```python
from build123d import *

# Parameters (mm, degrees)
CYLINDER1845_R     = 17
CYLINDER1845_DEPTH = 160
CYLINDER1789_R     = 4
CYLINDER1789_DEPTH = 100
CYLINDER1790_R     = 4
CYLINDER1790_DEPTH = 100
CYLINDER1809_R     = 1.5
CYLINDER1809_DEPTH = 100
CYLINDER1825_R     = 1.5
CYLINDER1825_DEPTH = 100
CYLINDER1824_R     = 1.5
CYLINDER1824_DEPTH = 100
CYLINDER1806_R     = 1.5
CYLINDER1806_DEPTH = 100
CYLINDER1805_R     = 1.5
CYLINDER1805_DEPTH = 100
CYLINDER1804_R     = 1.5
CYLINDER1804_DEPTH = 100
CYLINDER1803_R     = 1.5
CYLINDER1803_DEPTH = 100
CYLINDER1828_R     = 1.5
CYLINDER1828_DEPTH = 100
CYLINDER1826_R     = 4
CYLINDER1826_DEPTH = 100
CYLINDER1788_R     = 4
CYLINDER1788_DEPTH = 100
CYLINDER1787_R     = 4
CYLINDER1787_DEPTH = 100
CYLINDER1783_R     = 4
CYLINDER1783_DEPTH = 100
CYLINDER1785_R     = 4
CYLINDER1785_DEPTH = 100
CYLINDER1784_R     = 4
CYLINDER1784_DEPTH = 100
CYLINDER1786_R     = 4
CYLINDER1786_DEPTH = 100
CYLINDER1827_R     = 4
CYLINDER1827_DEPTH = 100
CYLINDER1797_R     = 4
CYLINDER1797_DEPTH = 20
CYLINDER1796_R     = 4
CYLINDER1796_DEPTH = 20
CYLINDER1795_R     = 4
CYLINDER1795_DEPTH = 20
CYLINDER1794_R     = 4
CYLINDER1794_DEPTH = 40
CYLINDER1793_R     = 4
CYLINDER1793_DEPTH = 40
CYLINDER1792_R     = 4
CYLINDER1792_DEPTH = 40
CYLINDER1791_R     = 4
CYLINDER1791_DEPTH = 40
CYLINDER1817_R     = 4
CYLINDER1817_DEPTH = 20
CYLINDER1798_R     = 59
CYLINDER1798_DEPTH = 16
CHAMFER061_SIZE    = 4
FILLET025_R        = 4


with BuildPart() as obj1:
    # Cylinder1845 → Cylinder1845 (new body)
    with BuildSketch(Plane(origin=(-18, 0, -60), x_dir=(1, 0, 0), z_dir=(0, 0, 1))):
        Circle(CYLINDER1845_R)
    extrude(amount=CYLINDER1845_DEPTH)


with BuildPart() as obj2:
    # Cylinder1789 → Cylinder1789 (new body)
    with BuildSketch(Plane(origin=(14, 0, -18), x_dir=(1, 0, 0), z_dir=(0, 0, 1))):
        Circle(CYLINDER1789_R)
    extrude(amount=CYLINDER1789_DEPTH)


with BuildPart() as obj3:
    # Cylinder1790 → Cylinder1790 (new body)
    with BuildSketch(Plane(origin=(90, 0, -18), x_dir=(1, 0, 0), z_dir=(0, 0, 1))):
        Circle(CYLINDER1790_R)
    extrude(amount=CYLINDER1790_DEPTH)

    # Compound957: union obj2
    add(obj2.part)


with BuildPart() as obj4:
    # Cylinder1809 → Cylinder1809 (new body)
    with BuildSketch(Plane(origin=(-34, -16, -60), x_dir=(1, 0, 0), z_dir=(0, 0, 1))):
        Circle(CYLINDER1809_R)
    extrude(amount=CYLINDER1809_DEPTH)


with BuildPart() as obj5:
    # Cylinder1825 → Cylinder1825 (new body)
    with BuildSketch(Plane(origin=(34, -16, -60), x_dir=(1, 0, 0), z_dir=(0, 0, 1))):
        Circle(CYLINDER1825_R)
    extrude(amount=CYLINDER1825_DEPTH)


with BuildPart() as obj6:
    # Cylinder1824 → Cylinder1824 (new body)
    with BuildSketch(Plane(origin=(34, 16, -60), x_dir=(1, 0, 0), z_dir=(0, 0, 1))):
        Circle(CYLINDER1824_R)
    extrude(amount=CYLINDER1824_DEPTH)


with BuildPart() as obj7:
    # Cylinder1806 → Cylinder1806 (new body)
    with BuildSketch(Plane(origin=(16, 34, -60), x_dir=(1, 0, 0), z_dir=(0, 0, 1))):
        Circle(CYLINDER1806_R)
    extrude(amount=CYLINDER1806_DEPTH)


with BuildPart() as obj8:
    # Cylinder1805 → Cylinder1805 (new body)
    with BuildSketch(Plane(origin=(10, -36, -60), x_dir=(1, 0, 0), z_dir=(0, 0, 1))):
        Circle(CYLINDER1805_R)
    extrude(amount=CYLINDER1805_DEPTH)


with BuildPart() as obj9:
    # Cylinder1804 → Cylinder1804 (new body)
    with BuildSketch(Plane(origin=(-16, -34, -60), x_dir=(1, 0, 0), z_dir=(0, 0, 1))):
        Circle(CYLINDER1804_R)
    extrude(amount=CYLINDER1804_DEPTH)


with BuildPart() as obj10:
    # Cylinder1803 → Cylinder1803 (new body)
    with BuildSketch(Plane(origin=(-16, 34, -60), x_dir=(1, 0, 0), z_dir=(0, 0, 1))):
        Circle(CYLINDER1803_R)
    extrude(amount=CYLINDER1803_DEPTH)


with BuildPart() as obj11:
    # Cylinder1828 → Cylinder1828 (new body)
    with BuildSketch(Plane(origin=(-34, 16, -60), x_dir=(1, 0, 0), z_dir=(0, 0, 1))):
        Circle(CYLINDER1828_R)
    extrude(amount=CYLINDER1828_DEPTH)

    # Compound954: union obj4, obj5, obj6, obj7, obj8, obj9, obj10
    add(obj4.part)
    add(obj5.part)
    add(obj6.part)
    add(obj7.part)
    add(obj8.part)
    add(obj9.part)
    add(obj10.part)


with BuildPart() as obj12:
    # Cylinder1826 → Cylinder1826 (new body)
    with BuildSketch(Plane(origin=(-16, 34, -90), x_dir=(1, 0, 0), z_dir=(0, 0, 1))):
        Circle(CYLINDER1826_R)
    extrude(amount=CYLINDER1826_DEPTH)


with BuildPart() as obj13:
    # Cylinder1788 → Cylinder1788 (new body)
    with BuildSketch(Plane(origin=(-16, -34, -90), x_dir=(1, 0, 0), z_dir=(0, 0, 1))):
        Circle(CYLINDER1788_R)
    extrude(amount=CYLINDER1788_DEPTH)


with BuildPart() as obj14:
    # Cylinder1787 → Cylinder1787 (new body)
    with BuildSketch(Plane(origin=(34, -16, -90), x_dir=(1, 0, 0), z_dir=(0, 0, 1))):
        Circle(CYLINDER1787_R)
    extrude(amount=CYLINDER1787_DEPTH)


with BuildPart() as obj15:
    # Cylinder1783 → Cylinder1783 (new body)
    with BuildSketch(Plane(origin=(16, 34, -90), x_dir=(1, 0, 0), z_dir=(0, 0, 1))):
        Circle(CYLINDER1783_R)
    extrude(amount=CYLINDER1783_DEPTH)


with BuildPart() as obj16:
    # Cylinder1785 → Cylinder1785 (new body)
    with BuildSketch(Plane(origin=(10, -36, -90), x_dir=(1, 0, 0), z_dir=(0, 0, 1))):
        Circle(CYLINDER1785_R)
    extrude(amount=CYLINDER1785_DEPTH)


with BuildPart() as obj17:
    # Cylinder1784 → Cylinder1784 (new body)
    with BuildSketch(Plane(origin=(-34, 16, -90), x_dir=(1, 0, 0), z_dir=(0, 0, 1))):
        Circle(CYLINDER1784_R)
    extrude(amount=CYLINDER1784_DEPTH)


with BuildPart() as obj18:
    # Cylinder1786 → Cylinder1786 (new body)
    with BuildSketch(Plane(origin=(34, 16, -90), x_dir=(1, 0, 0), z_dir=(0, 0, 1))):
        Circle(CYLINDER1786_R)
    extrude(amount=CYLINDER1786_DEPTH)


with BuildPart() as obj19:
    # Cylinder1827 → Cylinder1827 (new body)
    with BuildSketch(Plane(origin=(-34, -16, -90), x_dir=(1, 0, 0), z_dir=(0, 0, 1))):
        Circle(CYLINDER1827_R)
    extrude(amount=CYLINDER1827_DEPTH)

    # Compound956: union obj12, obj13, obj14, obj15, obj16, obj17, obj18
    add(obj12.part)
    add(obj13.part)
    add(obj14.part)
    add(obj15.part)
    add(obj16.part)
    add(obj17.part)
    add(obj18.part)


with BuildPart() as obj20:
    # Cylinder1797 → Cylinder1797 (new body)
    with BuildSketch(Plane(origin=(103, 12, -20), x_dir=(1, 0, 0), z_dir=(0, 0, 1))):
        Circle(CYLINDER1797_R)
    extrude(amount=CYLINDER1797_DEPTH)


with BuildPart() as obj21:
    # Cylinder1796 → Cylinder1796 (new body)
    with BuildSketch(Plane(origin=(76, 24, -18), x_dir=(1, 0, 0), z_dir=(0, 0, 1))):
        Circle(CYLINDER1796_R)
    extrude(amount=CYLINDER1796_DEPTH)


with BuildPart() as obj22:
    # Cylinder1795 → Cylinder1795 (new body)
    with BuildSketch(Plane(origin=(91, -27, -18), x_dir=(1, 0, 0), z_dir=(0, 0, 1))):
        Circle(CYLINDER1795_R)
    extrude(amount=CYLINDER1795_DEPTH)


with BuildPart() as obj23:
    # Cylinder1794 → Cylinder1794 (new body)
    with BuildSketch(Plane(origin=(13, -27, -18), x_dir=(1, 0, 0), z_dir=(0, 0, 1))):
        Circle(CYLINDER1794_R)
    extrude(amount=CYLINDER1794_DEPTH)


with BuildPart() as obj24:
    # Cylinder1793 → Cylinder1793 (new body)
    with BuildSketch(Plane(origin=(28, 24, -18), x_dir=(1, 0, 0), z_dir=(0, 0, 1))):
        Circle(CYLINDER1793_R)
    extrude(amount=CYLINDER1793_DEPTH)


with BuildPart() as obj25:
    # Cylinder1792 → Cylinder1792 (new body)
    with BuildSketch(Plane(origin=(1, -12, -18), x_dir=(1, 0, 0), z_dir=(0, 0, 1))):
        Circle(CYLINDER1792_R)
    extrude(amount=CYLINDER1792_DEPTH)


with BuildPart() as obj26:
    # Cylinder1791 → Cylinder1791 (new body)
    with BuildSketch(Plane(origin=(1, 12, -18), x_dir=(1, 0, 0), z_dir=(0, 0, 1))):
        Circle(CYLINDER1791_R)
    extrude(amount=CYLINDER1791_DEPTH)


with BuildPart() as obj27:
    # Cylinder1817 → Cylinder1817 (new body)
    with BuildSketch(Plane(origin=(103, -12, -20), x_dir=(1, 0, 0), z_dir=(0, 0, 1))):
        Circle(CYLINDER1817_R)
    extrude(amount=CYLINDER1817_DEPTH)

    # Compound955: union obj20, obj21, obj22, obj23, obj24, obj25, obj26
    add(obj20.part)
    add(obj21.part)
    add(obj22.part)
    add(obj23.part)
    add(obj24.part)
    add(obj25.part)
    add(obj26.part)


with BuildPart() as fillet025:
    # Cylinder1798 → Cylinder1798 (new body)
    with BuildSketch(Plane.XY.offset(2)):
        Circle(CYLINDER1798_R)
    extrude(amount=CYLINDER1798_DEPTH)

    # Cut614: cut obj27
    add(obj27.part, mode=Mode.SUBTRACT)

    # Cut615: cut obj19
    add(obj19.part, mode=Mode.SUBTRACT)

    # Cut619: cut obj11
    add(obj11.part, mode=Mode.SUBTRACT)

    # Chamfer061
    chamfer061_edges = [fillet025.edges().sort_by_distance(p)[0] for p in [
        (-59, 0, 2),
    ]]
    chamfer(chamfer061_edges, length=CHAMFER061_SIZE)

    # Cut620: cut obj3
    add(obj3.part, mode=Mode.SUBTRACT)


with BuildPart() as fillet025_1:
    # Cut620 placement: moved
    add(fillet025.part.moved(Location((-0.5, 0, 14))))

    # Cut613: cut obj1
    add(obj1.part, mode=Mode.SUBTRACT)

    # Fillet025
    fillet025_edges = [fillet025_1.edges().sort_by_distance(p)[0] for p in [
        (-35, 0, 32),
    ]]
    fillet(fillet025_edges, radius=FILLET025_R)


solid = fillet025_1.part
```
Model file for the job. Use its own axes, mm. A direction names the side the tool comes from. Give positions to 0.01 mm unless a question says otherwise; leave off trailing zeros. Use CSV: the item, a comma, the result in double quotes. Start each with the question number.
1) Flat gauge pins, fed straight in: pin 1 Ø1 at (y, z) = (-7.5, 20.5) entering from +X; pin 2 Ø5 at (x, z) = (-38.5, 23.5) entering from -Y; pin 3 Ø8 at (y, z) = (38, 27.5) entering from +X. Where does each tip first touch, or does it go through?
2) Slice it at A-A on y = 34. Give the number of separate pieces and of enclosed holes in the cut face, plus the area to 3 significant figures.
3) Mould opens along Y. For faces 1 (the flat face through (11, -11, 16)), 2 (the flat face through (-32.8, -15.9, 24)), 3 (the conical face through (52.145, 16.579, 16.194)) say: released by +Y, released by -Y, zero draft, split by the parting line, or undercut.
4) Tool access for faces 4 (the flat face through (9, -38, 24)), 5 (the cylindrical face through (-0.021, 15.966, 23.888)): list every direction of +Z, -Z, +X, -X, +Y, -Y with a clear straight run to the whole face (end or side of a thin tool).
5) Wall check: line 1 (Y direction, x = 0.5, z = 24); line 2 (X direction, y = -34, z = 20); line 3 (X direction, y = 34, z = 20.25). Give the ranges that are in metal, low to high.
Computed values:
1,pin 1,"stops at x = 58.08"
1,pin 2,"stops at y = -47.12"
1,pin 3,"stops at x = 47.72"
2,separate pieces,"3"
2,enclosed holes,"0"
2,area,"1,350 mm^2"
3,face 1,"zero draft"
3,face 2,"undercut"
3,face 3,"split by the parting line"
4,face 4,"-Z"
4,face 5,"+Z, -Z"
5,line 1,"y = -58.99 to -16, -8 to 8, 16 to 58.99"
5,line 2,"x = -48.72 to -20.5, -12.5 to 6.04, 12.96 to 47.72"
5,line 3,"x = -48.72 to -20.5, -12.5 to 11.5, 19.5 to 47.72"
